For this review, take the finished solid that the model builds, in its own axes (mm). Coordinates: 2 decimals unless noted, no trailing zeros. Loops run counter-clockwise (first coordinate to the right, second up) from the corner with the lowest first, then second, coordinate; pieces in that order, holes last. Notation, with made-up numbers: (-1.5, 12.5) -> (8.5, 12.5) arc R21 cw to (8.5, 43.5) -> close; hole circle Ø3 at (-31.75, -39.75). An arc over 180 degrees is marked (long way). One line per item, written item: value.
from build123d import *

# Parameters (mm, degrees)
F1_DEPTH = 25.4
F2_R     = 5.08


with BuildPart() as f1:
    # F0 (on Top) → F1 (new body)
    with BuildSketch(Plane.XY):
        Polygon((17.004497, 35.310201), (-17.004497, 35.310201), (-38.208757, 8.7209), (-30.641044, -24.435417), (0, -39.191367), (30.641044, -24.435417), (38.208757, 8.7209), align=None)
    extrude(amount=F1_DEPTH)

    # F2
    f2_edges = [f1.edges().sort_by_distance(p)[0] for p in [
        (15.320522, -31.813392, 25.4),
    ]]
    fillet(f2_edges, radius=F2_R)


solid = f1.part
1. Take a section at B-B, the plane y = 6. Give the boundary of the cut face in (x, z), and give its area (3 significant figures).
Return value:
outline: (-37.59, 0) -> (37.59, 0) -> (37.59, 25.4) -> (-37.59, 25.4) -> close
area: 1,910 mm2
2. Insertion check: pin 1 Ø8 at (x, z) = (7, 14.5) entering from -Y; pin 2 Ø10 at (y, z) = (21.5, 13.5) entering from -X; pin 3 Ø3 at (y, z) = (19, 12.5) entering from +X. Each pin has a flat end and moves straight along its axis. Give the tip position at first contact, or say it passes through.
Return value:
pin 1: stops at y = -37.75
pin 2: stops at x = -32.01
pin 3: stops at x = 31.21
3. Take a section at D-D, the plane x = -8. Give the boundary of the cut face in (y, z).
Return value:
outline: (-35.34, 0) -> (35.31, 0) -> (35.31, 25.4) -> (-35.34, 25.4) -> close
4. Take a section at C-C, the plane z = 22.75. Give the boundary of the cut face in (x, y).
Return value:
outline: (-38.21, 8.72) -> (-30.64, -24.44) -> (-0.71, -38.85) -> (30.82, -23.66) -> (38.21, 8.72) -> (17, 35.31) -> (-17, 35.31) -> close
5. To check wall thickness, follow probe 1 along X at (y, z) = (-9, 3); probe 2 along X at (y, z) = (30, 18); probe 3 along Y at (x, z) = (27, 7). State the ranges of each line that lie inside material, in increasing order. Write a range as from..to.
Return value:
probe 1: x = -34.16..34.16
probe 2: x = -21.24..21.24
probe 3: y = -26.19..22.78
6. Take a section at A-A, the plane z = 4. Give the boundary of the cut face in (x, y), and give its area (3 significant figures).
Return value:
outline: (-38.21, 8.72) -> (-30.64, -24.44) -> (0, -39.19) -> (30.64, -24.44) -> (38.21, 8.72) -> (17, 35.31) -> (-17, 35.31) -> close
area: 4,200 mm2
